Design review of the part built by this model. Coordinates are the model's own, in mm. Coordinates: 2 decimals unless noted, no trailing zeros. Loops run counter-clockwise (first coordinate to the right, second up) from the corner with the lowest first, then second, coordinate; pieces in that order, holes last. Notation, with made-up numbers: (12, 54) - (45, 54) arc R26 cw to (45, 85) - close; hole circle Ø5 at (2, -16). An arc over 180 degrees is marked (long way). Answer in a Markdown table with one row per item. Add a question column.
(1) To check wall thickness, follow L1, parallel to Z at x = -34.5, y = 0; L2, parallel to Y at x = -19, z = 36.5; L3, parallel to Z at x = -12, y = 14. State the ranges of each line that lie inside material, in increasing order. Write a range as [from, to].
(2) We need section B-B, the plane y = 0. Write out the cut boundary in (x, z) (1 decimal), plus the area to 3 significant figures.
(3) We need section C-C, the plane z = 64. Write out the cut boundary in (x, y).
(4) Clearance check with flat-ended pins moving along their axes: pin 1 (1 mm diameter, centred on x = -13.5, z = 36.5, fed in from +Y); pin 2 (8 mm diameter, centred on x = -6.5, z = 61, fed in from -Y); pin 3 (8 mm diameter, centred on x = -32, z = 28.5, fed in from -Y). State where each tip first meets the part, or that it passes through.
from build123d import *

# Parameters (mm, degrees)
F2_SIZE = 5.08


with BuildPart() as f1:
    # F0 (on Front) → F1 (revolve)
    with BuildSketch(Plane.XZ):
        with BuildLine():
            Line((-19.05, 0), (0, 0))
            Line((0, 0), (0, 13.886647))
            ThreePointArc((0, 13.886647), (-4.445, 18.331647), (0, 22.776647))
            Line((0, 22.776647), (0, 51.508222))
            ThreePointArc((0, 51.508222), (-4.441492, 55.949714), (0, 60.391206))
            Line((0, 60.391206), (0, 76.2))
            Line((0, 76.2), (-19.05, 76.2))
            Line((-19.05, 76.2), (-19.05, 0))
        make_face()
    revolve(axis=Axis((-19.05, 0, 38.1), (0, 0, -1)))

    # F2
    f2_edges = [f1.edges().sort_by_distance(p)[0] for p in [
        (-38.1, 0, 76.2),
        (-38.1, 0, 0),
    ]]
    chamfer(f2_edges, length=F2_SIZE)


solid = f1.part
Responses:
| question | item | result |
|---|---|---|
| 1 | L1 | z = [1.48, 15.72], [20.94, 53.35], [58.55, 74.72] |
| 1 | L2 | y = [-19.05, 19.05] |
| 1 | L3 | z = [1.7, 15.44], [21.22, 53.06], [58.84, 74.5] |
| 2 | outline | (-38.1, 5.1) - (-33, 0) - (-5.1, 0) - (0, 5.1) - (0, 13.9) arc R4.4 cw to (0, 22.8) - (0, 51.5) arc R4.4 cw to (0, 60.4) - (0, 71.1) - (-5.1, 76.2) - (-33, 76.2) - (-38.1, 71.1) - (-38.1, 60.4) arc R4.4 cw to (-38.1, 51.5) - (-38.1, 22.8) arc R4.4 cw to (-38.1, 13.9) - close |
| 2 | area | 2,730 mm2 |
| 3 | outline | circle Ø38.1 at (-19.05, 0) |
| 4 | pin 1 | stops at y = 18.37 |
| 4 | pin 2 | stops at y = -17.02 |
| 4 | pin 3 | stops at y = -16.82 |
